Source: CAD feature listing. Evaluate the final solid. Frame: model axes, mm. A direction names the side the tool comes from. Give positions to 0.01 mm unless a question says otherwise; leave off trailing zeros. Order: outer loops, then holes, each group sorted by start corner. A loop starts at its lowest first (then second) coordinate and runs counter-clockwise, first axis right, second up. Notation, with made-up numbers: (84, 4) -> (130, 4) arc R37 ccw to (130, 43) -> close; hole circle Ø2 at (51.25, 5.25). An arc over 180 degrees is marked (long way). Answer in a Markdown table with one row per item.
```python
from build123d import *

# Parameters (mm, degrees)
SKETCH_1_R      = 6.5
EXTRUDE_1_DEPTH = 6
CHAMFER_1_SIZE  = 2
CHAMFER_2_SIZE  = 1


with BuildPart() as part:
    # 草图1 → 凸台-拉伸1 (new, symmetric)
    with BuildSketch(Plane.XY):
        Polygon((-23, -14), (-23, 14), (-18, 14), (-18, 36), (0.696152423, 30.990381057), (18, 21), (18, -21), (0.696152423, -30.990381057), (-18, -36), (-18, -14), align=None)
        with Locations(Location((0, 0, 0), (0, 0, 180))):
            Circle(SKETCH_1_R, mode=Mode.SUBTRACT)
    extrude(amount=EXTRUDE_1_DEPTH, both=True)

    # 倒角1
    chamfer_1_edges = [part.edges().sort_by_distance(p)[0] for p in [
        (-8.651923789, -33.495190528, -6),
        (9.348076211, -25.995190528, -6),
        (9.348076211, 25.995190528, 6),
        (9.348076211, 25.995190528, -6),
        (-8.651923789, 33.495190528, -6),
        (9.348076211, -25.995190528, 6),
        (-8.651923789, -33.495190528, 6),
        (-8.651923789, 33.495190528, 6),
    ]]
    chamfer(chamfer_1_edges, length=CHAMFER_1_SIZE)

    # 倒角2
    chamfer_2_edges = [part.edges().sort_by_distance(p)[0] for p in [
        (6.5, 0, 6),
        (6.5, 0, -6),
    ]]
    chamfer(chamfer_2_edges, length=CHAMFER_2_SIZE)


solid = part.part
```
(1) Section query B-B (z = -1.25). Return the cut outline in (x, y).
A:
| item | result |
|---|---|
| outline | (-23, -14) -> (-18, -14) -> (-18, -36) -> (0.7, -30.99) -> (18, -21) -> (18, 21) -> (0.7, 30.99) -> (-18, 36) -> (-18, 14) -> (-23, 14) -> close; hole circle Ø13 at (0, 0) |
(2) Section query C-C (x = -15). Return the cut outline in (y, z).
A:
| item | result |
|---|---|
| outline | (-35.2, -4) -> (-33.13, -6) -> (33.13, -6) -> (35.2, -4) -> (35.2, 4) -> (33.13, 6) -> (-33.13, 6) -> (-35.2, 4) -> close |
(3) First-contact query: pin 1 Ø1.5 at (y, z) = (-23, 0) entering from +X; pin 2 Ø2 at (x, z) = (-17.5, -2) entering from -Y; pin 3 Ø3.5 at (y, z) = (-25.5, -1) entering from -X; pin 4 Ø2.5 at (x, z) = (-20, -0.5) entering from +Y. Flat tips, straight axial feed; report the tip coordinate or a pass-through.
A:
| item | result |
|---|---|
| pin 1 | stops at x = 15.83 |
| pin 2 | stops at y = -36 |
| pin 3 | stops at x = -18 |
| pin 4 | stops at y = 14 |
(4) Section query D-D (x = 9). Return the cut outline in (y, z).
A:
| item | result |
|---|---|
| outline | (-26.2, -4) -> (-23.89, -6) -> (23.89, -6) -> (26.2, -4) -> (26.2, 4) -> (23.89, 6) -> (-23.89, 6) -> (-26.2, 4) -> close |
(5) Section query A-A (y = 0). Return the cut outline in (x, z).
A:
| item | result |
|---|---|
| outline | (-23, -6) -> (-7.5, -6) -> (-6.5, -5) -> (-6.5, 5) -> (-7.5, 6) -> (-23, 6) -> close; (6.5, -5) -> (7.5, -6) -> (18, -6) -> (18, 6) -> (7.5, 6) -> (6.5, 5) -> close |
(6) Access query for faces 4 (the flat face through (-8.52, -33.46, 0.06)), 5 (the flat face through (-21, 14, 0)), 6 (the flat face through (-18, -25, 0)). Directions: +Z, -Z, +X, -X, +Y, -Y. A direction counts if a zero-diameter tool reaches every point of the face in a straight line with its end or side. Return the directions, or none.
A:
| item | result |
|---|---|
| face 4 | +Z, -Z, +X, -Y |
| face 5 | +Z, -Z, -X, +Y |
| face 6 | +Z, -Z, -X, -Y |
(7) Pull-direction query (Y, two-part tool) for faces 1 (the flat face through (18, 0, 0)), 2 (the cylindrical face through (5.158, 3.955, -0.07)), 3 (the flat face through (9.227, 24.927, 4.986)); classes: +Y half, -Y half, draft (parallel to the pull), parting line (faces both ways), or undercut.
A:
| item | result |
|---|---|
| face 1 | draft |
| face 2 | undercut |
| face 3 | +Y half |
(8) Ray query, probe 1 along X at (y, z) = (19, -3.75); probe 2 along Y at (x, z) = (0, -2); probe 3 along X at (y, z) = (2, 3). Return the intervals inside material, ascending.
A:
| item | result |
|---|---|
| probe 1 | x = -18 to 18 |
| probe 2 | y = -31.18 to -6.5, 6.5 to 31.18 |
| probe 3 | x = -23 to -6.18, 6.18 to 18 |
